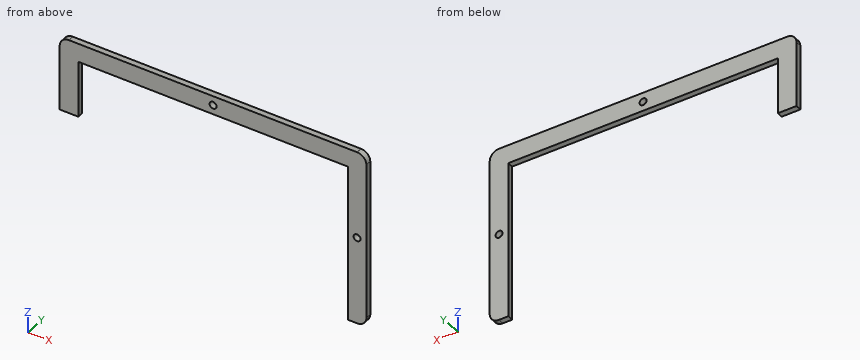
```python
from build123d import *

# Parameters (mm, degrees)
SKETCH1_R           = 1.875
BOSS_EXTRUDE1_DEPTH = 3.175


with BuildPart() as part:
    # Sketch1 → Boss-Extrude1 (new body)
    with BuildSketch(Plane(origin=(0, 0, 0), x_dir=(1, 0, 0), z_dir=(0, 1, 0))):
        with BuildLine():
            Line((-5, 0), (-160, 0))
            ThreePointArc((-160, 0), (-163.535533906, 1.464466094), (-165, 5))
            Line((-165, 5), (-165, 40.5))
            Line((-165, 40.5), (-155, 40.5))
            Line((-155, 40.5), (-155, 10))
            Line((-155, 10), (-10, 10))
            Line((-10, 10), (-10, 85))
            Line((-10, 85), (-10, 95))
            Line((-10, 95), (-5, 95))
            ThreePointArc((-5, 95), (-1.464466094, 93.535533906), (0, 90))
            Line((0, 90), (0, 5))
            ThreePointArc((0, 5), (-1.464466094, 1.464466094), (-5, 0))
        make_face()
        with Locations(Location((-5, 47.5, 0), (0, 0, 270))):
            Circle(SKETCH1_R, mode=Mode.SUBTRACT)
        with Locations(Location((-82.5, 5, 0), (0, 0, 270))):
            Circle(SKETCH1_R, mode=Mode.SUBTRACT)
    extrude(amount=BOSS_EXTRUDE1_DEPTH)


solid = part.part
```
Check sheet for the modelled part. Datum: model origin and axes. Units: mm. Coordinates: 2 decimals unless noted, no trailing zeros. Write each loop counter-clockwise with the first axis right and the second up, starting at its lowest first coordinate (ties: lowest second). Pieces come first, ordered by that corner, then holes. Notation, with made-up numbers: M 24,-5.75 L 72,-5.75 A24 cw 72,9.25 Z; hole C 12.25,84.25 d7. An arc over 180 degrees is marked long. Write item = value, one per line. Start each with the question number.
1. Sectioned sample at A-A (x = -82.5). Record the cut outline in (y, z) (3 decimals).
2. Go/stop test with flat-tipped pins: pin 1 (1.5 mm diameter, centred on x = -115.5, y = 2.5, fed in from -Z); pin 2 (1.5 mm diameter, centred on y = 3, z = -56.5, fed in from -X); pin 3 (4.5 mm diameter, centred on x = -82.5, z = -5, fed in from +Y) (3 decimals). Record where each tip stops, or that it passes through.
3. Thickness scan on probe 1 along X at (y, z) = (1.9, -5) (3 decimals); probe 2 along X at (y, z) = (1.95, -47.5) (3 decimals); probe 3 along X at (y, z) = (2.7, -70.5). Record the ranges inside material, lowest first.
4. Sectioned sample at D-D (x = -40). Record the cut outline in (y, z) (3 decimals), then the cut area to 4 significant figures.
5. Sectioned sample at C-C (y = 1.75). Record the cut outline in (x, z) (3 decimals), then the cut area to 3 significant figures.
6. Sectioned sample at B-B (z = -47.5). Record the cut outline in (x, y) (3 decimals).
The answers:
q1.outline = M 0,-10 L 3.175,-10 L 3.175,-6.875 L 0,-6.875 Z; M 0,-3.125 L 3.175,-3.125 L 3.175,0 L 0,0 Z
q2.pin_1 = -10
q2.pin_2 = -10
q2.pin_3 = 3.175
q3.probe_1 = -165 to -84.375, -80.625 to 0
q3.probe_2 = -10 to -6.875, -3.125 to 0
q3.probe_3 = -10 to 0
q4.outline = M 0,-10 L 3.175,-10 L 3.175,0 L 0,0 Z
q4.area = 31.75 mm²
q5.outline = M -165,-40.5 L -155,-40.5 L -155,-10 L -10,-10 L -10,-95 L -5,-95 A5 ccw 0,-90 L 0,-5 A5 ccw -5,0 L -160,0 A5 ccw -165,-5 Z; hole C -82.5,-5 d3.75; hole C -5,-47.5 d3.75
q5.area = 2,770 mm²
q6.outline = M -10,0 L -6.875,0 L -6.875,3.175 L -10,3.175 Z; M -3.125,0 L 0,0 L 0,3.175 L -3.125,3.175 Z
